Check sheet for the drawn part. Datum: minimum x, y, z corner. Units: mm. Round coordinates to 2 decimals unless told otherwise and drop trailing zeros.
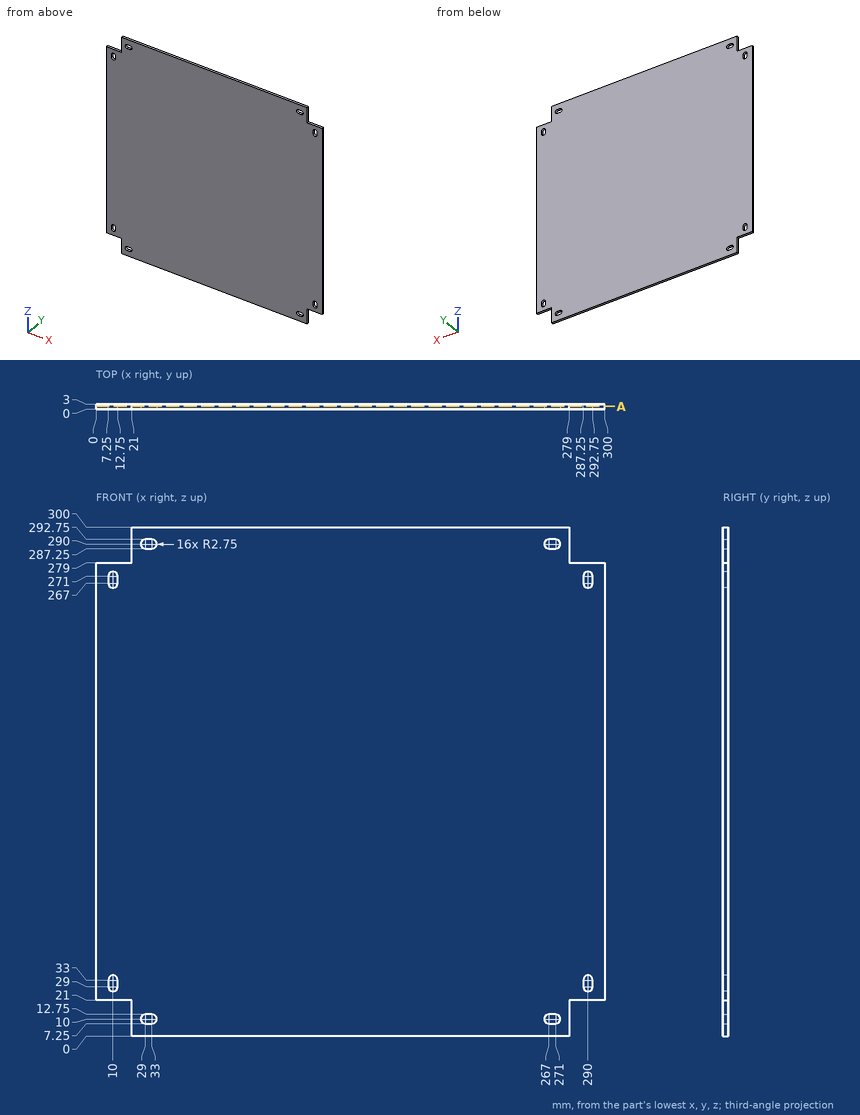
1. Scan lines: line 1 along Z through (x, y) = (29, 0.6); line 2 along X through (y, z) = (2.6, 16). Record each from-to range of solid material in increasing order.
2. Sectioned sample at A-A, the plane y = 1.55. Give the number of separate pieces and of enclosed holes in the cut face, plus the area to 3 significant figures.
3. Go/stop test with flat-tipped pins: pin 1 (1.5 mm diameter, centred on y = 1.5, z = 10, fed in from -X); pin 2 (1.5 mm diameter, centred on y = 1, z = 290, fed in from +X); pin 3 (1.5 mm diameter, centred on x = 5.5, y = 2, fed in from +Z). Record where each tip stops, or that it passes through.
Computed values:
1. line 1: z = 0 to 7.25, 12.75 to 287.25, 292.75 to 300
1. line 2: x = 21 to 279
2. separate pieces: 1
2. enclosed holes: 8
2. area: 87,900 mm2
3. pin 1: stops at x = 21
3. pin 2: stops at x = 279
3. pin 3: stops at z = 279
